Check sheet for the modelled part. Datum: model origin and axes. Units: mm. A direction names the side the tool comes from. Round coordinates to 2 decimals unless told otherwise and drop trailing zeros. Write each loop counter-clockwise with the first axis right and the second up, starting at its lowest first coordinate (ties: lowest second). Pieces come first, ordered by that corner, then holes.
Item 1: Set-up check for faces 1 (the flat face through (7.392, 5, 9)), 2 (the flat face through (16, 5, 35)), 3 (the cylindrical face through (4, 8, 1)): record each of +Z, -Z, +X, -X, +Y, -Y from which the full face is reachable in a straight line by a thin tool's end or side.
Item 2: Section check A-A, the plane y = 4.5. Record the cut outline in (x, z), plus the area to 3 significant figures.
Item 3: Release check for a two-part mould opening along Y. For faces 4 (the cylindrical face through (28, 2, 49)), 5 (the cylindrical face through (3.64, 7.48, 4.23)), 6 (the flat face through (24.128, 5, 41)) record: pulls with the +Y half, pulls with the -Y half, needs draft (parallel to the pull), parting line crosses it, or undercut.
Item 4: Material ranges on line 1 along X through (y, z) = (9, 38); line 2 along Z through (x, y) = (24.5, 7); line 3 along Z through (x, y) = (23, 4.5), recorded low to high.
Item 5: Section check B-B, the plane z = 47. Record the cut outline in (x, y).
Item 6: Depth check by flat-ended pin: pin 1 (6 mm diameter, centred on y = 7.5, z = 17, fed in from -X); pin 2 (1.5 mm diameter, centred on x = 28, y = 4, fed in from +Z). Enter the tip coordinate at first touch or a pass-through.
Item 7: Section check D-D, the plane y = 6.75. Record the cut outline in (x, z), plus the area to 3 significant figures.
Item 8: Section check C-C, the plane x = 18.5. Record the cut outline in (y, z), plus the area to 3 significant figures.
from build123d import *

# Parameters (mm, degrees)
BOSS_EXTRU_1_DEPTH      = 10
CONG_1_R                = 5
ESQUISSE2_R             = 2.5
ENL_V_MAT_EXTRU_1_DEPTH = 50


with BuildPart() as part:
    # Esquisse1 → Boss.-Extru.1 (new body)
    with BuildSketch(Plane(origin=(0, 0, 0), x_dir=(1, 0, 0), z_dir=(0, 1, 0))):
        Polygon((7.392201948, 0), (0, 0), (0, -50), (7.392201948, -50), (7.392201948, -35), (15.760023564, -35), (15.760023564, -15), (7.392201948, -15), align=None)
        Polygon((24.127845179, -15), (15.760023564, -15), (15.760023564, -35), (24.127845179, -35), (24.127845179, -50), (31.520047127, -50), (31.520047127, 0), (24.127845179, 0), align=None)
    extrude(amount=BOSS_EXTRU_1_DEPTH)

    # Congé1
    cong_1_edges = [part.edges().sort_by_distance(p)[0] for p in [
        (27.823946153, 0, 50),
        (3.696100974, 0, 50),
        (3.696100974, 10, 50),
        (27.823946153, 10, 50),
        (27.823946153, 10, 0),
        (27.823946153, 0, 0),
        (3.696100974, 0, 0),
        (3.696100974, 10, 0),
    ]]
    fillet(cong_1_edges, radius=CONG_1_R - 0.0001)  # a hair under: the kernel refuses the full size

    # Esquisse2 → Enlèv. mat.-Extru.1 (cut)
    with BuildSketch(Plane.ZY):
        with Locations((4.552174391, 5)):
            Circle(ESQUISSE2_R)
        with Locations((45.447825609, 5)):
            Circle(ESQUISSE2_R)
    extrude(amount=-ENL_V_MAT_EXTRU_1_DEPTH, mode=Mode.SUBTRACT)


solid = part.part
Values found:
1. face 1: -Z, +Y, -Y
1. face 2: +Z, +Y, -Y
1. face 3: -Z, +X, -X, +Y
2. outline: (0, 0.03) - (7.39, 0.03) - (7.39, 2.1) - (0, 2.1) - close; (0, 7) - (7.39, 7) - (7.39, 15) - (24.13, 15) - (24.13, 7) - (31.52, 7) - (31.52, 43) - (24.13, 43) - (24.13, 35) - (7.39, 35) - (7.39, 43) - (0, 43) - close; (0, 47.9) - (7.39, 47.9) - (7.39, 49.97) - (0, 49.97) - close; (24.13, 0.03) - (31.52, 0.03) - (31.52, 2.1) - (24.13, 2.1) - close; (24.13, 47.9) - (31.52, 47.9) - (31.52, 49.97) - (24.13, 49.97) - close
2. area: 928 mm2
3. face 4: pulls with the -Y half
3. face 5: undercut
3. face 6: needs draft
4. line 1: x = 0 to 7.39, 24.13 to 31.52
4. line 2: z = 0.42 to 3.05, 6.05 to 43.95, 46.95 to 49.58
4. line 3: z = 15 to 35
5. outline: (0, 0.42) - (7.39, 0.42) - (7.39, 3.04) - (0, 3.04) - close; (0, 6.96) - (7.39, 6.96) - (7.39, 9.58) - (0, 9.58) - close; (24.13, 0.42) - (31.52, 0.42) - (31.52, 3.04) - (24.13, 3.04) - close; (24.13, 6.96) - (31.52, 6.96) - (31.52, 9.58) - (24.13, 9.58) - close
6. pin 1: stops at x = 0
6. pin 2: stops at z = 49.99
7. outline: (0, 0.32) - (7.39, 0.32) - (7.39, 2.77) - (0, 2.77) - close; (0, 6.34) - (7.39, 6.34) - (7.39, 15) - (24.13, 15) - (24.13, 6.34) - (31.52, 6.34) - (31.52, 43.66) - (24.13, 43.66) - (24.13, 35) - (7.39, 35) - (7.39, 43.66) - (0, 43.66) - close; (0, 47.23) - (7.39, 47.23) - (7.39, 49.68) - (0, 49.68) - close; (24.13, 0.32) - (31.52, 0.32) - (31.52, 2.77) - (24.13, 2.77) - close; (24.13, 47.23) - (31.52, 47.23) - (31.52, 49.68) - (24.13, 49.68) - close
7. area: 959 mm2
8. outline: (0, 15) - (10, 15) - (10, 35) - (0, 35) - close
8. area: 200 mm2
